from build123d import *

# Parameters (mm, degrees)
SKETCH1_W               = 406.4
SKETCH1_H               = 25.4
BOSS_EXTRUDE1_DEPTH     = 6.35
SKETCH2_R               = 2.4892
CUT_EXTRUDE1_DEPTH      = 1
CUT_EXTRUDE1_DEPTH_BACK = 7.35
SKETCH3_R               = 2.378070279
SKETCH3_R_2             = 2.20737703
CUT_EXTRUDE2_DEPTH      = 7.35
SKETCH4_W               = 25.4
SKETCH4_H               = 6.35
CUT_EXTRUDE3_DEPTH      = 95.25


with BuildPart() as part:
    # Sketch1 → Boss-Extrude1 (new body)
    with BuildSketch(Plane(origin=(0, 0, 0), x_dir=(1, 0, 0), z_dir=(0, 1, 0))):
        with Locations((203.2, 12.7)):
            Rectangle(SKETCH1_W, SKETCH1_H)
    extrude(amount=BOSS_EXTRUDE1_DEPTH)

    # Sketch2 → Cut-Extrude1 (cut, two sides)
    with BuildSketch(Plane(origin=(0, 6.35, 0), x_dir=(1, 0, 0), z_dir=(0, 1, 0))) as cut_extrude1_sk:
        with Locations((381, 12.7)):
            Circle(SKETCH2_R)
        with Locations((355.6, 12.7)):
            Circle(SKETCH2_R)
        with Locations((330.2, 12.7)):
            Circle(SKETCH2_R)
        with Locations((304.8, 12.7)):
            Circle(SKETCH2_R)
        with Locations((279.4, 12.7)):
            Circle(SKETCH2_R)
        with Locations((254, 12.7)):
            Circle(SKETCH2_R)
        with Locations((228.6, 12.7)):
            Circle(SKETCH2_R)
        with Locations((203.2, 12.7)):
            Circle(SKETCH2_R)
        with Locations((177.8, 12.7)):
            Circle(SKETCH2_R)
        with Locations((152.4, 12.7)):
            Circle(SKETCH2_R)
        with Locations((127, 12.7)):
            Circle(SKETCH2_R)
        with Locations((101.6, 12.7)):
            Circle(SKETCH2_R)
    extrude(amount=CUT_EXTRUDE1_DEPTH, mode=Mode.SUBTRACT)
    extrude(cut_extrude1_sk.sketch, amount=-CUT_EXTRUDE1_DEPTH_BACK, mode=Mode.SUBTRACT)

    # Sketch3 → Cut-Extrude2 (cut, through all)
    with BuildSketch(Plane.XZ):
        with Locations((63.5, -12.7)):
            Circle(SKETCH3_R)
        with Locations((38.1, -12.7)):
            Circle(SKETCH3_R_2)
    extrude(amount=-CUT_EXTRUDE2_DEPTH, mode=Mode.SUBTRACT)

    # Sketch4 → Cut-Extrude3 (cut)
    with BuildSketch(Plane.ZY):
        with Locations((-12.7, 3.175)):
            Rectangle(SKETCH4_W, SKETCH4_H)
    extrude(amount=-CUT_EXTRUDE3_DEPTH, mode=Mode.SUBTRACT)


solid = part.part
Design review of the part built by this model. Coordinates are the model's own, in mm. Round coordinates to 2 decimals unless told otherwise and drop trailing zeros. Return JSON: item names as keys, results as strings. Group by question number.
Item 1: We need section A-A on y = 4. Give the number of separate pieces and of enclosed holes in the cut face, and give its area (3 significant figures).
Item 2: For probe 1 along Z at (x, y) = (254, 5), list the stretches that pass through material, from the lowest coordinate up. Write a range as [from, to].
Item 3: The part is to be moulded in two halves that separate along Z. For faces 1 (the face through (251.513, 3.219, -12.809)), 2 (the face through (249, 3, -25.4)), 3 (the face through (95.25, 3, -13)), say which applies: pulls with the +Z half, pulls with the -Z half, needs draft (parallel to the pull), parting line crosses it, or undercut.
Model answer:
{
 "1": {"separate pieces": "1", "enclosed holes": "12", "area": "7,670 mm²"},
 "2": {"probe 1": "z = [-25.4, -15.19], [-10.21, 0]"},
 "3": {"face 1": "undercut", "face 2": "pulls with the -Z half", "face 3": "needs draft"}
}
